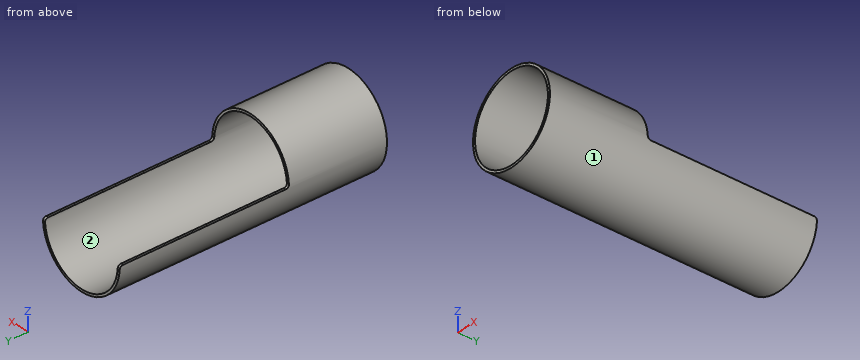
Autodesk Inventor part; units mm, degrees
ref_plane "YZ Plane" through (0, 0, 0) normal (1, 0, 0) x (0, 1, 0)
ref_plane "XZ Plane" through (0, 0, 0) normal (0, 1, 0) x (-1, 0, 0)
ref_plane "XY Plane" through (0, 0, 0) normal (0, 0, 1) x (1, 0, 0)
sketch "Boceto1" plane through (0, 0, 0) normal (0, 1, 0) x (-1, 0, 0)
  circle A0 centre (0, 0) radius 14.35
  circle A1 centre (0, 0) radius 15.15
  dimension "d0" = 28.7
  dimension "d1" = 0.8
extrude "Extrusión1" add sketch "Boceto1" along normal blind 90
sketch "Boceto2" plane through (0, 90, 0) normal (0, 1, 0) x (1, 0, 0)
  circle A0 centre (0, 0) radius 15.15
  circle A1 centre (0, 0) radius 14.35
  line L0 (-15.15, 0) -> (-14.35, 0)
  line L1 (14.35, 0) -> (15.15, 0)
extrude "Extrusión2" cut sketch "Boceto2" against normal blind 57 contours A0 L0 A1 L1 picked at (14.5976, -2.3533)
fillet "Empalme1" radius 1 4 edges at (-14.75, 33, 0) (14.75, 33, 0) (-14.75, 90, 0) (14.75, 90, 0)
properties part number "Embellecedor Espejo"
Model file for the job. Use its own axes, mm. Face numbers are marked on the shaded views. Coordinates: 2 decimals unless noted, no trailing zeros. Write each loop counter-clockwise with the first axis right and the second up, starting at its lowest first coordinate (ties: lowest second). Pieces come first, ordered by that corner, then holes. Notation, with made-up numbers: (26, 85.25) - (56, 85.25) arc R4 ccw to (56, 89.25) - close; hole circle Ø11 at (-11.75, 87.5). An arc over 180 degrees is marked (long way). One line per question, with ' | ' between items. Start each with the question number.
Q1. Cut at B-B, the plane z = 4. List the corners of the cut face in (x, y).
Q2. Pin check, flat tips, straight feed: pin 1 (0.9 mm diameter, centred on x = -15, y = 59.5, fed in from +Z); pin 2 (2 mm diameter, centred on x = -7, z = 9, fed in from +Y); pin 3 (2 mm diameter, centred on y = 39, z = 0.5, fed in from -X); pin 4 (11.5 mm diameter, centred on x = 1.5, z = 10, fed in from +Y). Stop position of each tip, or through.
Q3. Drill centre lines: line 1 (X direction, y = 21, z = 0); line 2 (Z direction, x = 0, y = 40). Where is each one in solid material? Low to high. Write a range as [from, to].
Q4. Cut at C-C, the plane y = 24. List the corners of the cut face in (x, z), then the cut area to 3 significant figures.
Q5. Cut at A-A, the plane x = 0. List the corners of the cut face in (y, z).
Q6. Pull direction X, two halves, no side cores. Call the marked faces 1 and 2: pulls with the +X half, pulls with the -X half, needs draft (parallel to the pull), parting line crosses it, or undercut.
Q7. Cut at D-D, the plane y = 53. List the corners of the cut face in (x, z).
Answer below:
1) outline: (-14.61, 0) - (-13.78, 0) - (-13.78, 33) - (-14.61, 33) - close; (13.78, 0) - (14.61, 0) - (14.61, 33) - (13.78, 33) - close
2) pin 1: z = 0 | pin 2: through | pin 3: x = -15.15 | pin 4: y = 33
3) line 1: [-15.15, -14.35], [14.35, 15.15] | line 2: [-15.15, -14.35]
4) outline: circle Ø30.3 at (0, 0); hole circle Ø28.7 at (0, 0) | area: 74.1 mm^2
5) outline: (0, -15.15) - (90, -15.15) - (90, -14.35) - (0, -14.35) - close; (0, 14.35) - (33, 14.35) - (33, 15.15) - (0, 15.15) - close
6) face 1: parting line crosses it | face 2: undercut
7) outline: (-15.15, 0) arc R15.15 ccw to (15.15, 0) - (14.35, 0) arc R14.35 cw to (-14.35, 0) - close
